CAD build for the part. Positions are in the model's coordinates, mm. Give positions to 0.01 mm unless a question says otherwise; leave off trailing zeros. Order: outer loops, then holes, each group sorted by start corner. A loop starts at its lowest first (then second) coordinate and runs counter-clockwise, first axis right, second up. Notation, with made-up numbers: (3.25, -2.75) -> (55.25, -2.75) arc R23 ccw to (55.25, 14.25) -> close; hole circle Ø1 at (30, 41). An arc over 180 degrees is marked (long way). Answer as CSV lines item,"result".
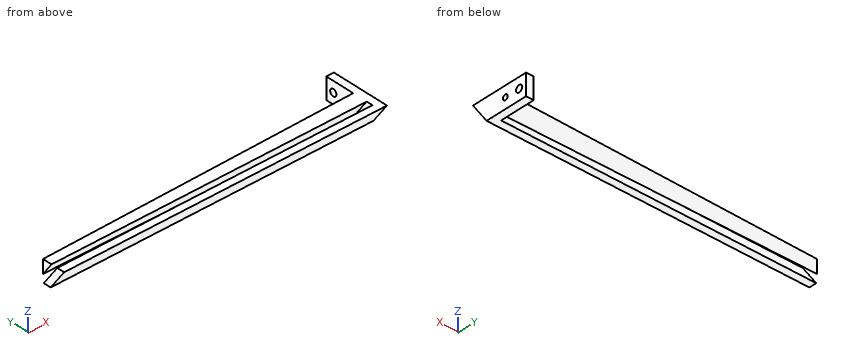
```python
from build123d import *

# Parameters (mm, degrees)
EXTRUDE_1_DEPTH     = 425
CUT_EXTRUDE_1_DEPTH = 425
SKETCH_4_R          = 4.5
SKETCH_4_R_2        = 3.5
CUT_EXTRUDE_2_DEPTH = 425
CUT_EXTRUDE_START   = -10
CUT_EXTRUDE_3_DEPTH = 415


with BuildPart() as part:
    # 草图1 → 凸台-拉伸1 (new body)
    with BuildSketch(Plane(origin=(0, 0, 0), x_dir=(0, 0, -1), z_dir=(1, 0, 0))):
        Polygon((-31.009476957, 41.355268582), (-3.009476957, 41.355268582), (-3.009476957, -15.744731418), (-31.009476957, -35.350542488), align=None)
    extrude(amount=EXTRUDE_1_DEPTH)

    # 草图2 → 切除-拉伸1 (cut)
    with BuildSketch(Plane.XY.offset(31.009476957)):
        Polygon((415, 41.355268582), (415, 2.555268582), (0, -4.688583363), (0, 41.355268582), align=None)
    extrude(amount=-CUT_EXTRUDE_1_DEPTH, mode=Mode.SUBTRACT)

    # 草图4 → 切除-拉伸2 (cut)
    with BuildSketch(Plane(origin=(425, 0, 0), x_dir=(0, 0, -1), z_dir=(1, 0, 0))):
        with Locations((-17.009476957, 31.355268582)):
            Circle(SKETCH_4_R)
        with Locations((-17.009476957, 11.355268582)):
            Circle(SKETCH_4_R_2)
    extrude(amount=-CUT_EXTRUDE_2_DEPTH, mode=Mode.SUBTRACT)

    # 草图6 → 切除-拉伸3 (cut)
    with BuildSketch(Plane(origin=(425, 0, 0), x_dir=(0, 0, -1), z_dir=(1, 0, 0)).offset(CUT_EXTRUDE_START)):
        Polygon((-31.009476957, -25.34019086), (-3.009476957, -5.73437979), (-3.009476957, 2.566887414), (-31.009476957, -17.038923656), align=None)
    extrude(amount=-CUT_EXTRUDE_3_DEPTH, mode=Mode.SUBTRACT)


solid = part.part
```
1) Band-saw the part on B-B, the plane z = 27.5. Write the cut outline in (x, y), then the cut area to 3 significant figures.
Data:
outline,"(0, -32.89) -> (425, -32.89) -> (425, 41.36) -> (415, 41.36) -> (415, 2.56) -> (0, -4.69) -> (0, -14.58) -> (415, -14.58) -> (415, -22.88) -> (0, -22.88) -> close"
area,"10,500 mm2"
2) Band-saw the part on D-D, the plane y = -29. Write the cut outline in (x, z), then the cut area to 3 significant figures.
Data:
outline,"(0, 21.94) -> (425, 21.94) -> (425, 31.01) -> (0, 31.01) -> close"
area,"3,850 mm2"
3) Band-saw the part on C-C, the plane x = 274.5. Write the cut outline in (y, z), then the cut area to 3 significant figures.
Data:
outline,"(-35.35, 31.01) -> (-15.74, 3.01) -> (-5.73, 3.01) -> (-25.34, 31.01) -> close; (-17.04, 31.01) -> (0.1, 6.53) -> (0.1, 31.01) -> close"
area,"490 mm2"
4) Wall check: line 1 along X through (y, z) = (-13, 21); line 2 along Y through (x, z) = (320.5, 11); line 3 along Y through (x, z) = (190, 23). Give the ranges that are in metal, low to high. Write a range as [from, to].
Data:
line 1,"x = [415, 425]"
line 2,"y = [-21.34, -11.33], [-3.03, 0.91]"
line 3,"y = [-29.74, -19.73], [-11.43, -1.37]"
5) Band-saw the part on A-A, the plane x = 109. Write the cut outline in (y, z), then the cut area to 3 significant figures.
Data:
outline,"(-35.35, 31.01) -> (-15.74, 3.01) -> (-5.73, 3.01) -> (-25.34, 31.01) -> close; (-17.04, 31.01) -> (-2.79, 10.65) -> (-2.79, 31.01) -> close"
area,"425 mm2"
6) Pin check, flat tips, straight feed: P1, Ø1, axis at x = 230, z = 6.5, coming from the -Y side; P2, Ø10.5, axis at y = 31.36, z = 17.01, coming from the -X side; P3, Ø6, axis at x = 351.5, z = 16, coming from the -Y side. Stop position of each tip, or through.
Data:
P1,"stops at y = -18.54"
P2,"stops at x = 415"
P3,"stops at y = -26.94"
